Read the model definition and answer for the solid it produces. Units are mm, in the model's axes. A direction names the side the tool comes from. Coordinates: 2 decimals unless noted, no trailing zeros. Write each loop counter-clockwise with the first axis right and the second up, starting at its lowest first coordinate (ties: lowest second). Pieces come first, ordered by that corner, then holes.
1) Find the intervals of material crossed by line 1 (Y direction, x = 16.5, z = 19.5); line 2 (X direction, y = -21, z = 106); line 3 (Z direction, x = 60, y = -16.5), in increasing order.
2) The part is cut by section C-C (y = -13). Determine the outline of the cut face in (x, z).
3) This flat-tipped pin is pushed along its axis until it touches: pin 1 Ø11 at (x, y) = (5, -14.5) entering from +Z. Where does it stop, or does it pass through?
4) The part is cut by section A-A (z = -56). Determine the outline of the cut face in (x, y), then the cut area to 3 significant figures.
5) The part is cut by section B-B (x = -89.5). Determine the outline of the cut face in (y, z).
6) Determine the mould class of faces 1 (the face through (0, -5.08, 16)), 2 (the face through (2, -4, 138.789)), 3 (the face through (0, 0, 13)) for opening direction Y: +Y half, -Y half, draft (parallel to the pull), parting line (faces both ways), or undercut.
7) Which of the six approach directions +Z, -Z, +X, -X, +Y, -Y give full straight-line access (tool end or side, diameter ignored) to faces 4 (the face through (0, -16, -115.211)), 5 (the face through (0, -26.67, 16))?
from build123d import *

# Parameters (mm, degrees)
F0_W     = 254
F0_H     = 254
F1_DEPTH = 31.75
F2_T     = -5.08
F3_SIZE  = 1.27
F4_R     = 6.35


with BuildPart() as f1:
    # F0 (on Front) → F1 (new body)
    with BuildSketch(Plane.XZ):
        with Locations((2.089877, 11.789044)):
            Rectangle(F0_W, F0_H)
    extrude(amount=F1_DEPTH)

    # F2
    f2_openings = [f1.faces().sort_by_distance(p)[0] for p in [
        (2.089877, -15.875, 138.789044),
    ]]
    offset(amount=F2_T, openings=f2_openings)

    # F3
    f3_edges = [f1.edges().sort_by_distance(p)[0] for p in [
        (2.089877, -31.75, 138.789044),
        (-124.910123, -15.875, 138.789044),
        (2.089877, 0, 138.789044),
        (129.089877, -15.875, 138.789044),
    ]]
    chamfer(f3_edges, length=F3_SIZE)

    # F4
    f4_edges = [f1.edges().sort_by_distance(p)[0] for p in [
        (129.089877, -15.875, -115.210956),
        (-124.910123, -15.875, -115.210956),
    ]]
    fillet(f4_edges, radius=F4_R)


solid = f1.part
Reported:
1. line 1: y = -31.75 to -26.67, -5.08 to 0
1. line 2: x = -124.91 to -119.83, 124.01 to 129.09
1. line 3: z = -115.21 to -110.13
2. outline: (-124.91, -108.86) arc R6.35 ccw to (-118.56, -115.21) - (122.74, -115.21) arc R6.35 ccw to (129.09, -108.86) - (129.09, 137.52) - (127.82, 138.79) - (124.01, 138.79) - (124.01, -110.13) - (-119.83, -110.13) - (-119.83, 138.79) - (-123.64, 138.79) - (-124.91, 137.52) - close
3. pin 1: stops at z = -110.13
4. outline: (-124.91, -31.75) - (129.09, -31.75) - (129.09, 0) - (-124.91, 0) - close; hole (-119.83, -26.67) - (124.01, -26.67) - (124.01, -5.08) - (-119.83, -5.08) - close
4. area: 2,800 mm2
5. outline: (-31.75, -115.21) - (0, -115.21) - (0, 137.52) - (-1.27, 138.79) - (-5.08, 138.79) - (-5.08, -110.13) - (-26.67, -110.13) - (-26.67, 138.79) - (-30.48, 138.79) - (-31.75, 137.52) - close
6. face 1: undercut
6. face 2: draft
6. face 3: +Y half
7. face 4: -Z, +X, -X, +Y, -Y
7. face 5: +Z
